Work out the finished part from the listing and answer in its coordinate system (mm). Coordinates: 2 decimals unless noted, no trailing zeros. Order: outer loops, then holes, each group sorted by start corner. A loop starts at its lowest first (then second) coordinate and runs counter-clockwise, first axis right, second up. Notation, with made-up numbers: (54.25, 30.5) - (67.25, 30.5) arc R10 cw to (67.25, 34.5) - close; hole circle Ø8 at (49.25, 20). An arc over 180 degrees is marked (long way). Answer as a JSON object with one key per item and string values. Group by question number.
1) Section A-A (x = -88.5) is taken. Give the vertices of the cut face in (y, z) (3 decimals), plus the area to 3 significant figures.
2) Section B-B (y = -7) is taken. Give the vertices of the cut face in (x, z) (3 decimals), plus the area to 3 significant figures.
3) Each of these flat-tipped pins is pushed along its axis until it touches: P1, Ø10, axis at x = -50.5, z = -18, coming from the -Y side (3 decimals); P2, Ø10, axis at x = 59.5, z = -20.5, coming from the +Y side (3 decimals); P3, Ø6.5, axis at y = 76, z = -21.5, coming from the +X side (3 decimals). Where does it stop, or does it pass through?
4) Find the intervals of material crossed by line 1 along X through (y, z) = (-79, -17.75) (3 decimals); line 2 along Y through (x, z) = (-73.5, -17.25) (3 decimals), in increasing order.
5) Section C-C (z = -18.75) is taken. Give the vertices of the cut face in (x, y) (3 decimals), plus the area to 3 significant figures.
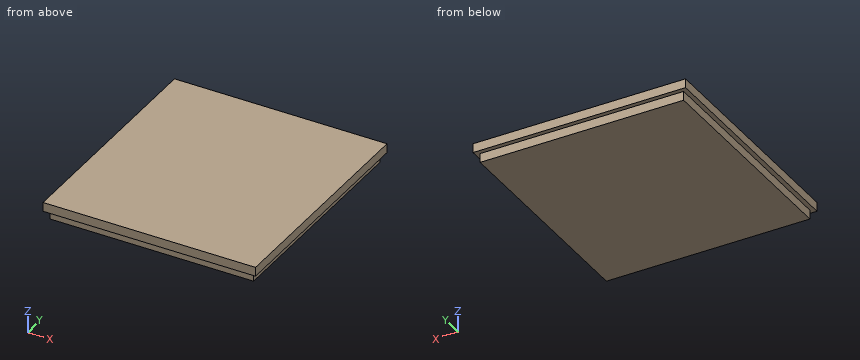
from build123d import *

# Parameters (mm, degrees)
F0_W     = 285.75
F0_H     = 311.15
F1_DEPTH = 25.4
F3_W     = 285.75
F3_H     = 12.7
F4_DEPTH = 6.35
F2_W     = 285.75
F2_H     = 12.7
F5_DEPTH = 6.35
F8_DEPTH = 6.35
F9_DEPTH = 6.35


with BuildPart() as f1:
    # F0 (on Top) → F1 (new body)
    with BuildSketch(Plane.XY):
        Rectangle(F0_W, F0_H)
    extrude(amount=-F1_DEPTH)

    # F3 (on face) → F4 (join)
    with BuildSketch(Plane(origin=(0, 155.575, 0), x_dir=(-1, 0, 0), z_dir=(0, 1, 0))):
        with Locations((0, -6.35)):
            Rectangle(F3_W, F3_H)
    extrude(amount=F4_DEPTH)

    # F2 (on face) → F5 (join)
    with BuildSketch(Plane.XZ.offset(155.575)):
        with Locations((0, -6.35)):
            Rectangle(F2_W, F2_H)
    extrude(amount=F5_DEPTH)

    # F7 (on face) → F8 (join)
    with BuildSketch(Plane(origin=(-142.875, 0, 0), x_dir=(0, -1, 0), z_dir=(-1, 0, 0))):
        Polygon((161.925, 0), (-161.925, 0), (-161.925, -12.7), (-155.575, -12.7), (155.575, -12.7), (161.925, -12.7), align=None)
    extrude(amount=F8_DEPTH)

    # F6 (on face) → F9 (join)
    with BuildSketch(Plane.YZ.offset(142.875)):
        Polygon((161.925, 0), (-161.925, 0), (-161.925, -12.7), (-155.575, -12.7), (155.575, -12.7), (161.925, -12.7), align=None)
    extrude(amount=F9_DEPTH)


solid = f1.part
Report:
{
 "1": {"outline": "(-161.925, -12.7) - (-155.575, -12.7) - (-155.575, -25.4) - (155.575, -25.4) - (155.575, -12.7) - (161.925, -12.7) - (161.925, 0) - (-161.925, 0) - close", "area": "8,060 mm²"},
 "2": {"outline": "(-149.225, -12.7) - (-142.875, -12.7) - (-142.875, -25.4) - (142.875, -25.4) - (142.875, -12.7) - (149.225, -12.7) - (149.225, 0) - (-149.225, 0) - close", "area": "7,420 mm²"},
 "3": {"P1": "stops at y = -155.575", "P2": "stops at y = 155.575", "P3": "stops at x = 142.875"},
 "4": {"line 1": "x = -142.875 to 142.875", "line 2": "y = -155.575 to 155.575"},
 "5": {"outline": "(-142.875, -155.575) - (142.875, -155.575) - (142.875, 155.575) - (-142.875, 155.575) - close", "area": "88,900 mm²"}
}
